Autodesk Inventor part; units mm, degrees
ref_plane "YZ Plane" through (0, 0, 0) normal (1, 0, 0) x (0, 1, 0)
ref_plane "XZ Plane" through (0, 0, 0) normal (0, 1, 0) x (-1, 0, 0)
ref_plane "XY Plane" through (0, 0, 0) normal (0, 0, 1) x (1, 0, 0)
sketch "Sketch1" plane through (0, 0, 0) normal (0, 1, 0) x (-1, 0, 0)
  line L0 (7.5, 80) -> (-7.5, 80)
  line L1 (-7.5, 80) -> (-7.5, -80)
  line L2 (-7.5, -80) -> (7.5, -80)
  line L3 (7.5, -80) -> (7.5, 80)
  line L4 (7.5, 80) -> (-7.5, -80) construction
  line L5 (7.5, -80) -> (-7.5, 80) construction
  line L6 (7.5, 75.75) -> (9, 75.75)
  line L7 (7.5, 80) -> (9, 80)
  line L8 (7.5, 71.5) -> (9, 71.5)
  arc A0 (9, 71.5) -> (9, 80) centre (9, 75.75) ccw
  line L9 (7.5, 74.6) -> (9, 74.6)
  line L10 (7.5, 76.9) -> (9, 76.9)
  arc A1 (9, 74.6) -> (9, 76.9) centre (9, 75.75) ccw
  line L11 (0, 80) -> (0, -80) construction
  line L12 (7.5, 0) -> (-7.5, 0) construction
  line L13 (-7.5, 75.75) -> (-9, 75.75)
  line L14 (-7.5, 80) -> (-9, 80)
  line L15 (-7.5, 71.5) -> (-9, 71.5)
  arc A2 (-9, 80) -> (-9, 71.5) centre (-9, 75.75) ccw
  line L16 (-7.5, 74.6) -> (-9, 74.6)
  line L17 (-7.5, 76.9) -> (-9, 76.9)
  arc A3 (-9, 76.9) -> (-9, 74.6) centre (-9, 75.75) ccw
  line L18 (7.5, -75.75) -> (9, -75.75)
  line L19 (7.5, -80) -> (9, -80)
  line L20 (7.5, -71.5) -> (9, -71.5)
  arc A4 (9, -80) -> (9, -71.5) centre (9, -75.75) ccw
  line L21 (7.5, -74.6) -> (9, -74.6)
  line L22 (7.5, -76.9) -> (9, -76.9)
  arc A5 (9, -76.9) -> (9, -74.6) centre (9, -75.75) ccw
  arc A6 (-9, -71.5) -> (-9, -80) centre (-9, -75.75) ccw
  line L23 (-7.5, -71.5) -> (-9, -71.5)
  line L24 (-7.5, -74.6) -> (-9, -74.6)
  arc A7 (-9, -74.6) -> (-9, -76.9) centre (-9, -75.75) ccw
  line L25 (-7.5, -75.75) -> (-9, -75.75)
  line L26 (-7.5, -76.9) -> (-9, -76.9)
  line L27 (-7.5, -80) -> (-9, -80)
  line L28 (7.5, 55) -> (27.5, 55)
  line L29 (32.5, 50) -> (32.5, 30)
  line L30 (32.5, 30) -> (42.5, 30)
  line L31 (47.5, 25) -> (47.5, 0)
  line L32 (64.2072, 0) -> (-38.11, 0) construction
  line L33 (7.5, -55) -> (27.5, -55)
  line L34 (32.5, -50) -> (32.5, -30)
  line L35 (32.5, -30) -> (42.5, -30)
  line L36 (47.5, -25) -> (47.5, 0)
  line L37 (27.5, 55) -> (32.5, 50)
  line L38 (42.5, 30) -> (47.5, 25)
  line L39 (47.5, -25) -> (42.5, -30)
  line L40 (32.5, -50) -> (27.5, -55)
  circle A8 centre (40.5, 0) radius 1.025
  circle A9 centre (-11.5, 0) radius 1.025
  line L41 (-7.5, 2.5) -> (-13.5, 2.5)
  line L42 (-13.5, 2.5) -> (-13.5, -2.5)
  line L43 (-13.5, -2.5) -> (-7.5, -2.5)
  line L44 (-7.5, -2.5) -> (-7.5, 2.5)
  point P0 (0, 0)
  point P1 (0, 0)
  point P2 (8.25, 71.5)
  point P3 (32.5, 55)
  point P4 (47.5, 30)
  point P5 (32.5, -55)
  point P6 (47.5, -30)
  dimension "d0" = 160
  dimension "d1" = 15
  dimension "d2" = 1.5
  dimension "d3" = 4.25
  dimension "d5" = 4.25
  dimension "d6" = 4.25
  dimension "d7" = 1.15
  dimension "d8" = 1.15
  dimension "d9" = 1.15
  dimension "d10" = 25
  dimension "d11" = 25
  dimension "d12" = 15
  dimension "d13" = 25
  dimension "d14" = 25
  dimension "d15" = 5
  dimension "d16" = 5
  dimension "d17" = 5
  dimension "d18" = 5
  dimension "d19" = 5
  dimension "d20" = 5
  dimension "d21" = 5
  dimension "d22" = 5
  dimension "d24" = 2.05
  dimension "d25" = 7
  dimension "d26" = 2.05
  dimension "d27" = 4
  dimension "d28" = 2.5
  dimension "d29" = 2.5
  dimension "d30" = 6
extrude "Extrusion1" add sketch "Sketch1" along normal blind 1.5 contours L3 L2 L1 L0 | L7 A0 L8 L3 L9 A1 L10 | L1 L17 A3 L16 L15 A2 L14 | L28 L37 L29 L30 L38 L31 L36 L39 L35 L34 L40 L33 L3 | L1 L43 L42 L41 | L20 A4 L19 L3 L22 A5 L21 | L1 L24 A7 L26 L27 A6 L23 | A9
properties part number "linefollower_chassy_model_3"
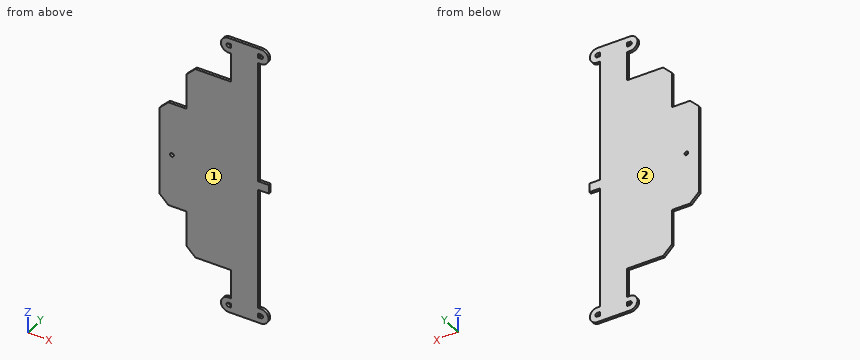
Here's how the part is built. I have some questions about the finished solid (model axes, mm). Face numbers are marked on the shaded views. Round coordinates to 2 decimals unless told otherwise and drop trailing zeros. Order: outer loops, then holes, each group sorted by start corner. A loop starts at its lowest first (then second) coordinate and runs counter-clockwise, first axis right, second up. Notation, with made-up numbers: M -36.75,86.5 L -27.75,86.5 A21 ccw -27.75,97.5 Z; hole C -19,62.25 d8. An arc over 180 degrees is marked long. Return JSON: item names as keys, results as strings. Group by question number.
1. If we section it at C-C on y = 0.65: State how many separate pieces and enclosed holes the cut face has, then the cut area to 3 significant figures.
2. I'm going to push a flat-ended pin straight in: pin 1 Ø0.8 at (y, z) = (1, -76) entering from +X. Where does the tip first touch, or does it pass through?
3. Please list where these lines run through material, in increasing order: probe 1 along Z at (x, y) = (-40.5, 1) (3 decimals); probe 2 along Z at (x, y) = (-17, 0.6); probe 3 along Z at (x, y) = (-10.5, 0.55).
4. If we section it at A-A on x = -17.5: List the corners of the cut face in (y, z) for me.
5. If we section it at B-B on z = 60.5: List the corners of the cut face in (x, y) for me.
6. If we mould it in two halves opening along Y, with no side actions, what happens to the marked faces 1 and 2? For each: pulls with the +Y half, pulls with the -Y half, needs draft (parallel to the pull), parting line crosses it, or undercut.
Reply:
{
 "1": {"separate pieces": "1", "enclosed holes": "5", "area": "6,170 mm^2"},
 "2": {"pin 1": "x = 13.25"},
 "3": {"probe 1": "-30 to -1.025, 1.025 to 30", "probe 2": "-55 to 55", "probe 3": "-79.73 to -71.77, -55 to 55, 71.77 to 79.73"},
 "4": {"outline": "M 0,-55 L 1.5,-55 L 1.5,55 L 0,55 Z"},
 "5": {"outline": "M -7.5,0 L 7.5,0 L 7.5,1.5 L -7.5,1.5 Z"},
 "6": {"face 1": "pulls with the -Y half", "face 2": "pulls with the +Y half"}
}
